Could you check a few things on this model? Use its own coordinates, in mm. A direction names the side the tool comes from. Round coordinates to 2 decimals unless told otherwise and drop trailing zeros. Loops run counter-clockwise (first coordinate to the right, second up) from the corner with the lowest first, then second, coordinate; pieces in that order, holes last. Notation, with made-up numbers: (-20, 79.25) -> (38, 79.25) arc R20 cw to (38, 103.25) -> close; hole circle Ø7 at (-35.5, 19.5). An arc over 180 degrees is marked (long way). Write each question's results on one line, items separated by ' | '. Start each with the question number.
1) Imagine slicing it at C-C, the plane y = -16. List the corners of the cut face in (x, z) for me.
2) Imagine slicing it at D-D, the plane z = 3.5. List the corners of the cut face in (x, y) for me, plus the area to 3 significant figures.
3) If I drill on probe 1 along X at (y, z) = (-9.5, 3); probe 2 along X at (y, z) = (-7.5, 17); probe 3 along Z at (x, y) = (34, -45.5), over which ranges is the centre line in solid material (lowest first)?
4) For P1, Ø10, axis at x = 60, y = -45, coming from the +Z side; P2, Ø1.1, axis at y = -49.5, z = 23.5, coming from the -X side; P3, Ø1.9, axis at x = -69, z = 19, coming from the -Y side, each with a flat end and sliding along its axis, tell me the tip position at first contact or that it passes through.
5) Which directions (+Z, -Z, +X, -X, +Y, -Y) give clear straight access to the entire face, cutting with the end or side of a thin tool? Please do faces 1 (the flat face through (66, 43, 14.5)), 2 (the flat face through (-59, -44.2, 12)), 3 (the flat face through (-69, 30.7, 12)).
6) Imagine slicing it at B-B, the plane x = -54.5. List the corners of the cut face in (y, z) for me, plus the area to 4 significant figures.
7) Imagine slicing it at A-A, the plane z = 22.5. List the corners of the cut face in (x, y) for me, plus the area to 3 significant figures.
8) We'd pull the mould along X, two halves only. Please class faces 4 (the flat face through (-69, -10, 21)), 5 (the flat face through (71.7, 1, 8)), 6 (the flat face through (-59, 44.2, 12)): pulls with the +X half, pulls with the -X half, needs draft (parallel to the pull), parting line crosses it, or undercut.
from build123d import *

# Parameters (mm, degrees)
SKETCH2_W                 = 143.4
SKETCH2_H                 = 101.4
BOSS_EXTRUDE2_DEPTH       = 10
SKETCH3_W                 = 121.8
SKETCH3_H                 = 85.8
CUT_EXTRUDE1_DEPTH        = 89.382011744
BOSS_EXTRUDE4_DEPTH       = 4.5
SKETCH8_W                 = 6.2
SKETCH8_H                 = 20
SKETCH8_W_2               = 10
SKETCH8_H_2               = 2.25
BOSS_EXTRUDE5_DEPTH       = 21.3
CUT_EXTRUDE3_REACH        = 130.072
SKETCH10_W                = 4.5
SKETCH10_H                = 4
MIRROR2_COPY_1_DEPTH      = 4.5
MIRROR2_COPY_2_SKETCH_W   = 6.2
MIRROR2_COPY_2_SKETCH_H   = 20
MIRROR2_COPY_2_SKETCH_W_2 = 10
MIRROR2_COPY_2_SKETCH_H_2 = 2.25
MIRROR2_COPY_2_DEPTH      = 21.3
MIRROR2_COPY_3_REACH      = 130.072
MIRROR2_COPY_3_SKETCH_W   = 4.5
MIRROR2_COPY_3_SKETCH_H   = 4
MIRROR2_COPY_4_DEPTH      = 4.5
MIRROR2_COPY_5_REACH      = 130.072
MIRROR2_COPY_5_SKETCH_W   = 4.5
MIRROR2_COPY_5_SKETCH_H   = 4


with BuildPart() as part:
    # Sketch2 → Boss-Extrude2 (new body)
    with BuildSketch(Plane.XY):
        Rectangle(SKETCH2_W, SKETCH2_H)
    extrude(amount=BOSS_EXTRUDE2_DEPTH)

    # Sketch3 → Cut-Extrude1 (cut, through all)
    with BuildSketch(Plane.XY.offset(10)):
        Rectangle(SKETCH3_W, SKETCH3_H)
    extrude(amount=-CUT_EXTRUDE1_DEPTH, mode=Mode.SUBTRACT)

    # Sketch6 → Boss-Extrude4 (add)
    with BuildSketch(Plane.XY.offset(10)):
        Polygon((51.7, 50.7), (51.7, 44.2), (65.7, 44.2), (65.7, 30.7), (71.7, 30.7), (71.7, 50.7), align=None)
    boss_extrude4 = extrude(amount=BOSS_EXTRUDE4_DEPTH)

    # Sketch8 → Boss-Extrude5 (add)
    with BuildSketch(Plane.XY.offset(10)):
        with Locations((68.6, 0)):
            Rectangle(SKETCH8_W, SKETCH8_H)
        with Locations((0, 49.575)):
            Rectangle(SKETCH8_W_2, SKETCH8_H_2)
    boss_extrude5 = extrude(amount=BOSS_EXTRUDE5_DEPTH)

    # Sketch10 → Cut-Extrude3 (cut, up to next)
    with BuildSketch(Plane(origin=(0, 50.7, 0), x_dir=(1, 0, 0), z_dir=(0, 1, 0)), mode=Mode.PRIVATE) as cut_extrude3_sk1:
        with Locations((0, -26.8)):
            Rectangle(SKETCH10_W, SKETCH10_H)
    cut_extrude3_tool1 = extrude(cut_extrude3_sk1.sketch, amount=-CUT_EXTRUDE3_REACH, mode=Mode.PRIVATE) & part.part
    cut_extrude3 = cut_extrude3_tool1.solids().sort_by_distance((0, 50.7, 26.8))[0]
    add(cut_extrude3, mode=Mode.SUBTRACT)

    # Mirror1: Boss-Extrude4, Boss-Extrude5, Cut-Extrude3 across plane
    add(boss_extrude4.mirror(Plane.ZX))
    add(boss_extrude5.mirror(Plane.ZX))
    add(cut_extrude3.mirror(Plane.ZX), mode=Mode.SUBTRACT)

    # Mirror2: Boss-Extrude5 across plane
    add(boss_extrude5.mirror(Plane(origin=(0, 0, 0), x_dir=(0, 0, 1), z_dir=(1, 0, 0))))

    # Mirror2 copy 1 sketch → Mirror2 copy 1 (add)
    with BuildSketch(Plane(origin=(0, 0, 10), x_dir=(-1, 0, 0), z_dir=(0, 0, 1))):
        Polygon((51.7, 50.7), (51.7, 44.2), (65.7, 44.2), (65.7, 30.7), (71.7, 30.7), (71.7, 50.7), align=None)
    extrude(amount=MIRROR2_COPY_1_DEPTH)

    # Mirror2 copy 2 sketch → Mirror2 copy 2 (add)
    with BuildSketch(Plane(origin=(0, 0, 10), x_dir=(-1, 0, 0), z_dir=(0, 0, 1))):
        with Locations((68.6, 0)):
            Rectangle(MIRROR2_COPY_2_SKETCH_W, MIRROR2_COPY_2_SKETCH_H)
        with Locations((0, 49.575)):
            Rectangle(MIRROR2_COPY_2_SKETCH_W_2, MIRROR2_COPY_2_SKETCH_H_2)
    extrude(amount=MIRROR2_COPY_2_DEPTH)

    # Mirror2 copy 3 sketch → Mirror2 copy 3 (cut, up to next)
    with BuildSketch(Plane(origin=(0, -50.7, 0), x_dir=(-1, 0, 0), z_dir=(0, -1, 0)), mode=Mode.PRIVATE) as mirror2_copy_3_sk1:
        with Locations((0, -26.8)):
            Rectangle(MIRROR2_COPY_3_SKETCH_W, MIRROR2_COPY_3_SKETCH_H)
    mirror2_copy_3_tool1 = extrude(mirror2_copy_3_sk1.sketch, amount=-MIRROR2_COPY_3_REACH, mode=Mode.PRIVATE) & part.part
    add(mirror2_copy_3_tool1.solids().sort_by_distance((0, -50.7, 26.8))[0], mode=Mode.SUBTRACT)

    # Mirror2 copy 4 sketch → Mirror2 copy 4 (add)
    with BuildSketch(Plane(origin=(0, 0, 10), x_dir=(-1, 0, 0), z_dir=(0, 0, 1))):
        Polygon((51.7, -50.7), (51.7, -44.2), (65.7, -44.2), (65.7, -30.7), (71.7, -30.7), (71.7, -50.7), align=None)
    extrude(amount=MIRROR2_COPY_4_DEPTH)

    # Mirror2 copy 5 sketch → Mirror2 copy 5 (cut, up to next)
    with BuildSketch(Plane(origin=(0, 50.7, 0), x_dir=(-1, 0, 0), z_dir=(0, 1, 0)), mode=Mode.PRIVATE) as mirror2_copy_5_sk1:
        with Locations((0, 26.8)):
            Rectangle(MIRROR2_COPY_5_SKETCH_W, MIRROR2_COPY_5_SKETCH_H)
    mirror2_copy_5_tool1 = extrude(mirror2_copy_5_sk1.sketch, amount=-MIRROR2_COPY_5_REACH, mode=Mode.PRIVATE) & part.part
    add(mirror2_copy_5_tool1.solids().sort_by_distance((0, 50.7, 26.8))[0], mode=Mode.SUBTRACT)


solid = part.part
Checked values:
1) outline: (-71.7, 0) -> (-60.9, 0) -> (-60.9, 10) -> (-71.7, 10) -> close; (60.9, 0) -> (71.7, 0) -> (71.7, 10) -> (60.9, 10) -> close
2) outline: (-71.7, -50.7) -> (71.7, -50.7) -> (71.7, 50.7) -> (-71.7, 50.7) -> close; hole (-60.9, -42.9) -> (60.9, -42.9) -> (60.9, 42.9) -> (-60.9, 42.9) -> close | area: 4,090 mm^2
3) probe 1: -71.7 to -60.9, 60.9 to 71.7 | probe 2: -71.7 to -65.5, 65.5 to 71.7 | probe 3: 0 to 10
4) P1: z = 14.5 | P2: x = -5 | P3: y = -10
5) face 1: +Z, +X, +Y | face 2: +Z | face 3: +Z, +X, -X
6) outline: (-50.7, 0) -> (-42.9, 0) -> (-42.9, 10) -> (-44.2, 10) -> (-44.2, 14.5) -> (-50.7, 14.5) -> close; (42.9, 0) -> (50.7, 0) -> (50.7, 14.5) -> (44.2, 14.5) -> (44.2, 10) -> (42.9, 10) -> close | area: 214.5 mm^2
7) outline: (-71.7, -10) -> (-65.5, -10) -> (-65.5, 10) -> (-71.7, 10) -> close; (-5, -50.7) -> (5, -50.7) -> (5, -48.45) -> (-5, -48.45) -> close; (-5, 48.45) -> (5, 48.45) -> (5, 50.7) -> (-5, 50.7) -> close; (65.5, -10) -> (71.7, -10) -> (71.7, 10) -> (65.5, 10) -> close | area: 293 mm^2
8) face 4: needs draft | face 5: pulls with the +X half | face 6: undercut
